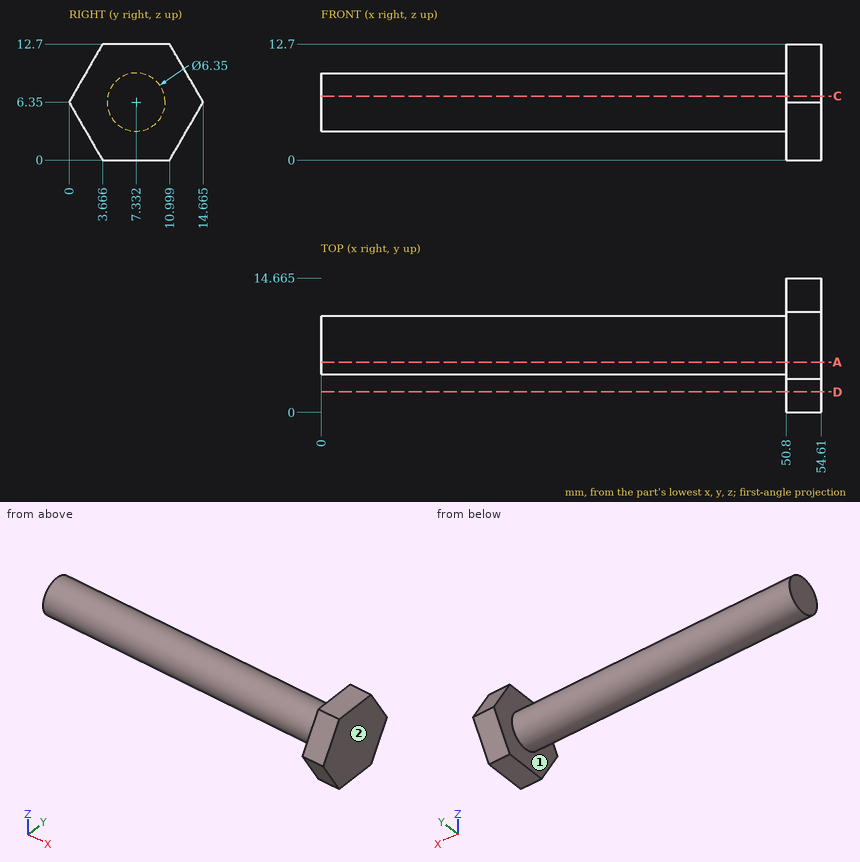
Answer from the drawing. Dimensions are ordinates in mm from the lowest x, y and z of the part. A direction names the side the tool comes from. Give positions to 0.01 mm unless a question says otherwise; leave off trailing zeros. Loops run counter-clockwise (first coordinate to the right, second up) from the corner with the lowest first, then second, coordinate; pieces in that order, holes last. Notation, with made-up numbers: (-4.5, -29.75) - (39.5, -29.75) arc R28 ccw to (39.5, -4.75) - close; hole circle Ø11 at (43.5, 52.25). An arc over 180 degrees is marked (long way). Answer as CSV lines item,"result". Start each with the question number.
Item 1: Find the intervals of material crossed by line 1 (X direction, y = 12, z = 10); line 2 (Y direction, x = 13.5, z = 6.25) (1 decimal); line 3 (Y direction, x = 49, z = 3.75) (1 decimal), in increasing order. Write a range as from..to.
Item 2: For the marked faces 1 and 2, determine the directions among +Z, -Z, +X, -X, +Y, -Y from which every point of the face is accessible in a straight line to the end or side of a thin tool.
Item 3: A cutting plane is placed at C-C on z = 7. Determine the outline of the cut face in (x, y) (1 decimal), then the cut area to 3 significant figures.
Item 4: Each of these flat-tipped pins is pushed along its axis until it touches: pin 1 (6 mm diameter, centred on x = 41.5, y = 10.5, fed in from +Z); pin 2 (5 mm diameter, centred on x = 38.5, y = 6, fed in from -Z) (3 decimals); pin 3 (4 mm diameter, centred on x = 29.5, z = 9.5, fed in from -Y). Where does it stop, or does it pass through?
Item 5: A cutting plane is placed at A-A on y = 5.5. Determine the outline of the cut face in (x, z), then the cut area to 3 significant figures.
Item 6: A cutting plane is placed at D-D on y = 2.25. Determine the outline of the cut face in (x, z), then the cut area to 3 significant figures.
Found:
1,line 1,"x = 50.8..54.61"
1,line 2,"y = 4.2..10.5"
1,line 3,"y = 5.5..9.2"
2,face 1,"-X"
2,face 2,"+Z, -Z, +X, +Y, -Y"
3,outline,"(0, 4.2) - (50.8, 4.2) - (50.8, 0.4) - (54.6, 0.4) - (54.6, 14.3) - (50.8, 14.3) - (50.8, 10.4) - (0, 10.4) - close"
3,area,"369 mm^2"
4,pin 1,"stops at z = 9.52"
4,pin 2,"stops at z = 3.175"
4,pin 3,"stops at y = 4.37"
5,outline,"(0, 3.76) - (50.8, 3.76) - (50.8, 0) - (54.61, 0) - (54.61, 12.7) - (50.8, 12.7) - (50.8, 8.94) - (0, 8.94) - close"
5,area,"312 mm^2"
6,outline,"(50.8, 2.45) - (54.61, 2.45) - (54.61, 10.25) - (50.8, 10.25) - close"
6,area,"29.7 mm^2"
